Read the model definition and answer for the solid it produces. Units are mm, in the model's axes. A direction names the side the tool comes from. Round coordinates to 2 decimals unless told otherwise and drop trailing zeros. Order: outer loops, then holes, each group sorted by start corner. A loop starts at its lowest first (then second) coordinate and runs counter-clockwise, first axis right, second up. Notation, with made-up numbers: (-36.5, -15.5) - (-0.5, -15.5) arc R24 cw to (-0.5, 22.5) - close; hole circle Ø4 at (-21.75, -25.75). An arc over 180 degrees is marked (long way). Put each result on its own line as item: value. Start each with the question number.
Q1. Section B-B on y = 0.3 is taken. Give the vertices of the cut face in (x, z) (3 decimals), then the cut area to 3 significant figures.
Q2. Section D-D on y = 1.45 is taken. Give the vertices of the cut face in (x, z) (3 decimals), then the cut area to 3 significant figures.
Q3. Section A-A on z = 0 is taken. Give the vertices of the cut face in (x, y) (3 decimals), then the cut area to 3 significant figures.
Q4. Find the intervals of material crossed by line 1 along X through (y, z) = (0.8, -0.1); line 2 along Z through (x, y) = (-2.5, 1.95); line 3 along Y through (x, z) = (2.5, 2.35), in increasing order. Write a range as from..to.
Q5. Each of these flat-tipped pins is pushed along its axis until it touches: pin 1 Ø0.8 at (x, z) = (2, 2.5) entering from +Y; pin 2 Ø2 at (x, z) = (-3.5, 2) entering from -Y. Where does it stop, or does it pass through?
Q6. Section C-C on x = 1.75 is taken. Give the vertices of the cut face in (y, z) (3 decimals), then the cut area to 3 significant figures.
Q7. Which of the six approach directions +Z, -Z, +X, -X, +Y, -Y give full straight-line access (tool end or side, diameter ignored) to faces 1 (the face through (-1, 2, 1.651)), 2 (the face through (-4.826, 1.611, 0.036)), 3 (the face through (2, 1.27, 2))?
from build123d import *

# Parameters (mm, degrees)
BOSS_EXTRUDE1_DEPTH = 3.175
SKETCH2_W           = 2.032
SKETCH2_H           = 1.524
SKETCH2_H_2         = 1.27
BOSS_EXTRUDE2_DEPTH = 1.27
CHAMFER1_SIZE       = 0.508
FILLET1_R           = 0.508


with BuildPart() as part:
    # Sketch1 → Boss-Extrude1 (new body)
    with BuildSketch(Plane(origin=(0, 0, 0), x_dir=(1, 0, 0), z_dir=(0, 1, 0))):
        with BuildLine():
            Line((-3.175, 1.651), (3.175, 1.651))
            ThreePointArc((3.175, 1.651), (4.826, 0), (3.175, -1.651))
            Line((3.175, -1.651), (-3.175, -1.651))
            ThreePointArc((-3.175, -1.651), (-4.826, 0), (-3.175, 1.651))
        make_face()
    extrude(amount=BOSS_EXTRUDE1_DEPTH)

    # Sketch2 → Boss-Extrude2 (add)
    with BuildSketch(Plane.XZ):
        with Locations((1.778, 2.413)):
            Rectangle(SKETCH2_W, SKETCH2_H)
        with Locations((-4.826, 0)):
            Rectangle(SKETCH2_W, SKETCH2_H_2)
    extrude(amount=-BOSS_EXTRUDE2_DEPTH)

    # Chamfer1
    chamfer1_edges = [part.edges().sort_by_distance(p)[0] for p in [
        (4.826, 3.175, 0),
        (0, 3.175, -1.651),
        (-4.826, 3.175, 0),
        (0, 3.175, 1.651),
    ]]
    chamfer(chamfer1_edges, length=CHAMFER1_SIZE)

    # Fillet1
    # the kernel refuses this fillet: 0.508 mm, written as the material it adds along each edge
    with BuildSketch(Plane(origin=(0.762, 0, 1.651), x_dir=(-1, 0, 0), z_dir=(0, 1, 0))) as fillet1_piece_1:
        with BuildLine():
            CenterArc((FILLET1_R, FILLET1_R), FILLET1_R, 180, 90)
            Line((0, FILLET1_R), (0, 0))
            Line((0, 0), (FILLET1_R, 0))
        make_face()
    extrude(amount=1.27)
    with BuildSketch(Plane(origin=(2.794, 0, 1.651), x_dir=(0.999982123617744, 0, -0.005979334824793291), z_dir=(0, 1, 0))) as fillet1_piece_2:
        with BuildLine():
            CenterArc((0.504975771, -0.507289957), FILLET1_R, 93.029693992, 86.627713317)
            Line((-0.003015148, -0.504252455), (-0.05381424, -0.503948704))
            Line((-0.05381424, -0.503948704), (-0.050799092, 0.00030375))
            Line((-0.050799092, 0.00030375), (0.00030375, 0.050799092))
            ThreePointArc((0.00030375, 0.050799092), (0.381296939, 0.048520965), (0.475441237, 0.050728996))
            Line((0.475441237, 0.050728996), (0.478126194, 0))
        make_face()
    extrude(amount=1.27)
    with BuildSketch(Plane(origin=(-4.699, 1.27, -0.635), x_dir=(0.45853775751047177, 0, -0.8886749264704544), z_dir=(0, -1, 0))) as fillet1_piece_3:
        with BuildLine():
            CenterArc((0.310391456, -0.506311404), FILLET1_R, 94.672926901, 58.034281249)
            Line((-0.141055407, -0.273374223), (0, 0))
            ThreePointArc((0, 0), (0.134502964, -0.005487936), (0.269005928, 0))
        make_face()
    extrude(amount=1.27)
    with BuildSketch(Plane(origin=(-4.699, 1.27, 0.635), x_dir=(0.45853775751047327, 0, 0.8886749264704539), z_dir=(0, -1, 0))) as fillet1_piece_4:
        with BuildLine():
            CenterArc((0.310391456, 0.506311404), FILLET1_R, 207.292791849, 58.034281249)
            Line((-0.141055407, 0.273374223), (0, 0))
            ThreePointArc((0, 0), (0.134502964, 0.005487936), (0.269005928, 0))
        make_face()
    extrude(amount=1.27)
    # the kernel refuses this fillet: 0.508 mm, written as the material it takes off along each edge
    with BuildSketch(Plane(origin=(0.762, -1.27, 3.175), x_dir=(0, 0, -1), z_dir=(0, 1, 0)), Plane(origin=(2.794, -1.27, 3.175), x_dir=(-1, 0, 0), z_dir=(0, 1, 0)), Plane(origin=(-5.842, -1.27, 0.635), x_dir=(0, 0, -1), z_dir=(0, 1, 0))) as fillet1_2_piece_1:
        with BuildLine():
            CenterArc((FILLET1_R, -FILLET1_R), FILLET1_R, 90, 90)
            Line((0, -FILLET1_R), (0, 0))
            Line((0, 0), (FILLET1_R, 0))
        make_face()
    extrude(amount=3.81, mode=Mode.SUBTRACT)
    with BuildSketch(Plane(origin=(-5.842, -1.27, -0.635), x_dir=(0, 0, 1), z_dir=(0, 1, 0))) as fillet1_2_piece_2:
        with BuildLine():
            CenterArc((FILLET1_R, FILLET1_R), FILLET1_R, 180, 90)
            Line((0, FILLET1_R), (0, 0))
            Line((0, 0), (FILLET1_R, 0))
        make_face()
    extrude(amount=3.81, mode=Mode.SUBTRACT)


solid = part.part
Findings:
1. outline: (-5.842, -0.127) arc R0.508 ccw to (-5.334, -0.635) - (-5.007, -0.635) arc R0.508 cw to (-4.576, -0.874) arc R1.651 ccw to (-3.175, -1.651) - (3.175, -1.651) arc R1.651 ccw to (3.272, 1.648) arc R0.508 cw to (2.794, 2.155) - (2.794, 2.667) arc R0.508 ccw to (2.286, 3.175) - (1.27, 3.175) arc R0.508 ccw to (0.762, 2.667) - (0.762, 2.159) arc R0.508 cw to (0.254, 1.651) - (-3.175, 1.651) arc R1.651 ccw to (-4.576, 0.874) arc R0.508 cw to (-5.007, 0.635) - (-5.334, 0.635) arc R0.508 ccw to (-5.842, 0.127) - close
1. area: 33.9 mm2
2. outline: (-3.175, -1.651) - (3.175, -1.651) arc R1.651 ccw to (3.175, 1.651) - (-3.175, 1.651) arc R1.651 ccw to start
2. area: 29.5 mm2
3. outline: (-5.842, 0) - (4.826, 0) - (4.826, 2.667) - (4.318, 3.175) - (-4.318, 3.175) - (-4.826, 2.667) - (-4.826, 1.27) - (-5.842, 1.27) - close
3. area: 31.7 mm2
4. line 1: -5.84..4.82
4. line 2: -1.65..1.65
4. line 3: 0..1.27
5. pin 1: y = 1.27
5. pin 2: y = 0
6. outline: (0, -1.651) - (2.667, -1.651) - (3.175, -1.143) - (3.175, 1.143) - (2.667, 1.651) - (1.27, 1.651) - (1.27, 3.175) - (0, 3.175) - close
6. area: 12.2 mm2
7. face 1: +Z, -X, +Y
7. face 2: -X, +Y
7. face 3: +Z, +X, -X, +Y
